Source: CAD feature listing. Evaluate the final solid. Frame: model axes, mm. Face numbers are marked on the shaded views. A direction names the side the tool comes from. Coordinates: 2 decimals unless noted, no trailing zeros. Order: outer loops, then holes, each group sorted by start corner. A loop starts at its lowest first (then second) coordinate and runs counter-clockwise, first axis right, second up. Notation, with made-up numbers: (22.5, -10.75) -> (74.5, -10.75) arc R20 ccw to (74.5, -3.75) -> close; hole circle Ø5 at (48, -15.5). An arc over 180 degrees is marked (long way). Put each result on its own line as item: value.
from build123d import *

# Parameters (mm, degrees)
SKETCH1_W           = 38.1
SKETCH1_H           = 38.1
SKETCH1_R           = 1.2
SKETCH1_R_2         = 7.5
SKETCH1_W_2         = 11
SKETCH1_H_2         = 5
BOSS_EXTRUDE1_DEPTH = 2.5
SKETCH1_6_R         = 7.5
BOSS_EXTRUDE2_DEPTH = 26.1


with BuildPart() as part:
    # Sketch1 → Boss-Extrude1 (new body)
    with BuildSketch(Plane(origin=(0, 0, 0), x_dir=(1, 0, 0), z_dir=(0, 1, 0))):
        Rectangle(SKETCH1_W, SKETCH1_H)
        with Locations((-14, -14)):
            Circle(SKETCH1_R, mode=Mode.SUBTRACT)
        with Locations((14, -14)):
            Circle(SKETCH1_R, mode=Mode.SUBTRACT)
        with Locations((14, 14)):
            Circle(SKETCH1_R, mode=Mode.SUBTRACT)
        with Locations((-14, 14)):
            Circle(SKETCH1_R, mode=Mode.SUBTRACT)
        Circle(SKETCH1_R_2, mode=Mode.SUBTRACT)
        with Locations((4.45, 13.35)):
            Rectangle(SKETCH1_W_2, SKETCH1_H_2, mode=Mode.SUBTRACT)
    extrude(amount=BOSS_EXTRUDE1_DEPTH)

    # Sketch1<6> → Boss-Extrude2 (add)
    with BuildSketch(Plane(origin=(0, 0, 0), x_dir=(1, 0, 0), z_dir=(0, 1, 0))):
        Circle(SKETCH1_6_R)
    extrude(amount=BOSS_EXTRUDE2_DEPTH)


solid = part.part
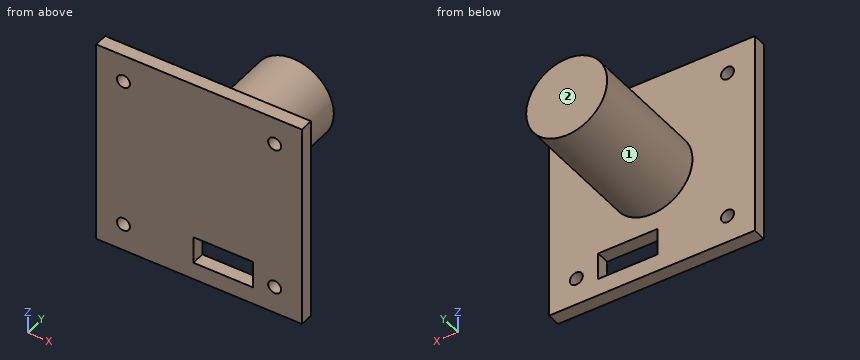
1. First-contact query: pin 1 (5 mm diameter, centred on x = 10.5, y = 15.5, fed in from +Z); pin 2 (2 mm diameter, centred on y = 23, z = -3, fed in from +X); pin 3 (1.5 mm diameter, centred on x = 0, y = 4, fed in from -Z); pin 4 (8 mm diameter, centred on y = 16.5, z = -10, fed in from -X). Flat tips, straight axial feed; report the tip coordinate or a pass-through.
Numbers:
pin 1: passes through
pin 2: stops at x = 7.23
pin 3: stops at z = -7.5
pin 4: stops at x = -4.5
2. Cut plane D-D on z = -12. Output: boundary loops of the cut face in (x, y), plus the area to 4 significant figures.
Numbers:
outline: (-19.05, 0) -> (-1.05, 0) -> (-1.05, 2.5) -> (-19.05, 2.5) -> close; (9.95, 0) -> (19.05, 0) -> (19.05, 2.5) -> (9.95, 2.5) -> close
area: 67.75 mm2
3. Cut plane C-C on x = 0. Output: boundary loops of the cut face in (y, z).
Numbers:
outline: (0, -19.05) -> (2.5, -19.05) -> (2.5, -15.85) -> (0, -15.85) -> close; (0, -10.85) -> (2.5, -10.85) -> (2.5, -7.5) -> (26.1, -7.5) -> (26.1, 7.5) -> (2.5, 7.5) -> (2.5, 19.05) -> (0, 19.05) -> close
4. Cut plane B-B on x = 14. Output: boundary loops of the cut face in (y, z), plus the area to 4 significant figures.
Numbers:
outline: (0, -19.05) -> (2.5, -19.05) -> (2.5, -15.2) -> (0, -15.2) -> close; (0, -12.8) -> (2.5, -12.8) -> (2.5, 12.8) -> (0, 12.8) -> close; (0, 15.2) -> (2.5, 15.2) -> (2.5, 19.05) -> (0, 19.05) -> close
area: 83.25 mm2
5. Set-up query: the marked faces 1 and 2. Return all of +Z, -Z, +X, -X, +Y, -Y with unobstructed straight access to the full face (end or side cutting, diameter ignored); none if empty.
Numbers:
face 1: +Y
face 2: +Z, -Z, +X, -X, +Y
6. Cut plane A-A on z = 14. Output: boundary loops of the cut face in (x, y), plus the area to 4 significant figures.
Numbers:
outline: (-19.05, 0) -> (-15.2, 0) -> (-15.2, 2.5) -> (-19.05, 2.5) -> close; (-12.8, 0) -> (12.8, 0) -> (12.8, 2.5) -> (-12.8, 2.5) -> close; (15.2, 0) -> (19.05, 0) -> (19.05, 2.5) -> (15.2, 2.5) -> close
area: 83.25 mm2
7. Ray query, line 1 along X through (y, z) = (0.5, -14); line 2 along Z through (x, y) = (14, 0.8). Return the intervals inside material, ascending.
Numbers:
line 1: x = -19.05 to -15.2, -12.8 to -1.05, 9.95 to 12.8, 15.2 to 19.05
line 2: z = -19.05 to -15.2, -12.8 to 12.8, 15.2 to 19.05
